from build123d import *

# Parameters (mm, degrees)
F0_W     = 127
F0_H     = 457.2
F1_DEPTH = 18.25625
F2_R     = 6.35
F2_R_2   = 3.175
F3_DEPTH = 15.875


with BuildPart() as f1:
    # F0 (on Top) → F1 (new body)
    with BuildSketch(Plane.XY):
        Rectangle(F0_W, F0_H)
    extrude(amount=F1_DEPTH)

    # F2 (on face) → F3 (cut)
    with BuildSketch(Plane.XY.offset(18.25625)):
        with Locations((47.625, 206.375)):
            Circle(F2_R)
        with Locations((-47.625, 206.375)):
            Circle(F2_R_2)
        with Locations((47.625, 174.625)):
            Circle(F2_R)
        with Locations((47.625, 142.875)):
            Circle(F2_R)
        with Locations((47.625, 111.125)):
            Circle(F2_R)
        with Locations((47.625, 79.375)):
            Circle(F2_R)
        with Locations((47.625, 47.625)):
            Circle(F2_R)
        with Locations((47.625, 15.875)):
            Circle(F2_R)
        with Locations((47.625, -15.875)):
            Circle(F2_R)
        with Locations((47.625, -47.625)):
            Circle(F2_R)
        with Locations((47.625, -79.375)):
            Circle(F2_R)
        with Locations((47.625, -111.125)):
            Circle(F2_R)
        with Locations((47.625, -142.875)):
            Circle(F2_R)
        with Locations((47.625, -174.625)):
            Circle(F2_R)
        with Locations((47.625, -206.375)):
            Circle(F2_R)
        with Locations((15.875, 206.375)):
            Circle(F2_R)
        with Locations((15.875, 174.625)):
            Circle(F2_R)
        with Locations((15.875, 142.875)):
            Circle(F2_R)
        with Locations((15.875, 111.125)):
            Circle(F2_R)
        with Locations((15.875, 79.375)):
            Circle(F2_R)
        with Locations((15.875, 47.625)):
            Circle(F2_R)
        with Locations((15.875, 15.875)):
            Circle(F2_R)
        with Locations((15.875, -15.875)):
            Circle(F2_R)
        with Locations((15.875, -47.625)):
            Circle(F2_R)
        with Locations((15.875, -79.375)):
            Circle(F2_R)
        with Locations((15.875, -111.125)):
            Circle(F2_R)
        with Locations((15.875, -142.875)):
            Circle(F2_R)
        with Locations((15.875, -174.625)):
            Circle(F2_R)
        with Locations((15.875, -206.375)):
            Circle(F2_R)
        with Locations((-47.625, 174.625)):
            Circle(F2_R_2)
        with Locations((-47.625, 142.875)):
            Circle(F2_R_2)
        with Locations((-47.625, 111.125)):
            Circle(F2_R_2)
        with Locations((-47.625, 79.375)):
            Circle(F2_R_2)
        with Locations((-47.625, 47.625)):
            Circle(F2_R_2)
        with Locations((-47.625, 15.875)):
            Circle(F2_R_2)
        with Locations((-47.625, -15.875)):
            Circle(F2_R_2)
        with Locations((-47.625, -47.625)):
            Circle(F2_R_2)
        with Locations((-47.625, -79.375)):
            Circle(F2_R_2)
        with Locations((-47.625, -111.125)):
            Circle(F2_R_2)
        with Locations((-47.625, -142.875)):
            Circle(F2_R_2)
        with Locations((-47.625, -174.625)):
            Circle(F2_R_2)
        with Locations((-47.625, -206.375)):
            Circle(F2_R_2)
        with Locations((-15.875, 206.375)):
            Circle(F2_R_2)
        with Locations((-15.875, 174.625)):
            Circle(F2_R_2)
        with Locations((-15.875, 142.875)):
            Circle(F2_R_2)
        with Locations((-15.875, 111.125)):
            Circle(F2_R_2)
        with Locations((-15.875, 79.375)):
            Circle(F2_R_2)
        with Locations((-15.875, 47.625)):
            Circle(F2_R_2)
        with Locations((-15.875, 15.875)):
            Circle(F2_R_2)
        with Locations((-15.875, -15.875)):
            Circle(F2_R_2)
        with Locations((-15.875, -47.625)):
            Circle(F2_R_2)
        with Locations((-15.875, -79.375)):
            Circle(F2_R_2)
        with Locations((-15.875, -111.125)):
            Circle(F2_R_2)
        with Locations((-15.875, -142.875)):
            Circle(F2_R_2)
        with Locations((-15.875, -174.625)):
            Circle(F2_R_2)
        with Locations((-15.875, -206.375)):
            Circle(F2_R_2)
    extrude(amount=-F3_DEPTH, mode=Mode.SUBTRACT)


solid = f1.part
Design review of the part built by this model. Coordinates are the model's own, in mm. A direction names the side the tool comes from. Coordinates: 2 decimals unless noted, no trailing zeros. Put each result on its own line as item: value.
1) Insertion check: P1, Ø1.9, axis at x = -47.5, y = -78.5, coming from the +Z side. The pin has a flat end and moves straight along its axis. Give the tip position at first contact, or say it passes through.
Response values:
P1: stops at z = 2.38
2) Take a section at A-A, the plane z = 7.5. Count the separate pieces of the cut face and the enclosed holes in it, and give its area (3 significant figures).
Response values:
separate pieces: 1
enclosed holes: 56
area: 53,600 mm²
3) Tool access review of faces 1 (the face through (15.05, 180.92, 10.43)), 2 (the face through (-1, 228.6, 9)): name each direction out of +Z, -Z, +X, -X, +Y, -Y from which nothing blocks a thin tool from reaching the whole face with its end or side.
Response values:
face 1: +Z
face 2: +Z, -Z, +X, -X, +Y
4) Wall thickness on L1, parallel to X at y = 43.5, z = 13.75; L2, parallel to X at y = 14.5, z = 8.25; L3, parallel to X at y = -43, z = 17.5: over which ranges is each line inside the solid? List them lowest first. Write a range as from..to.
Response values:
L1: x = -63.5..11.05, 20.7..42.8, 52.45..63.5
L2: x = -63.5..-50.49, -44.76..-18.74, -13.01..9.68, 22.07..41.43, 53.82..63.5
L3: x = -63.5..11.52, 20.23..43.27, 51.98..63.5
